Geometry check sheet. Reference: the model listing, model coordinates, mm. A direction names the side the tool comes from. Give positions to 0.01 mm unless a question says otherwise; leave off trailing zeros. Write each loop counter-clockwise with the first axis right and the second up, starting at its lowest first coordinate (ties: lowest second). Pieces come first, ordered by that corner, then holes. Notation, with made-up numbers: (-2, -16) - (26, -16) arc R31 ccw to (26, 21) - close; hole circle Ø7 at (69, 22.5). An arc over 180 degrees is marked (long way). Use a Markdown table: item, result.
```python
from build123d import *

# Parameters (mm, degrees)
SKETCH_1_R      = 20.5
EXTRUDE_1_DEPTH = 20
SKETCH_4_R      = 20
EXTRUDE_4_DEPTH = 28
SKETCH_2_R      = 11
EXTRUDE_2_DEPTH = 6
SKETCH_3_R      = 40
EXTRUDE_3_DEPTH = 5


with BuildPart() as part:
    # 草图1 → 凸台-拉伸1 (new body)
    with BuildSketch(Plane.XY):
        Circle(SKETCH_1_R)
    extrude(amount=EXTRUDE_1_DEPTH)

    # 草图4 → 凸台-拉伸4 (add)
    with BuildSketch(Plane.XY.offset(20)):
        Circle(SKETCH_4_R)
    extrude(amount=EXTRUDE_4_DEPTH)

    # 草图2 → 凸台-拉伸2 (add)
    with BuildSketch(Plane.XY.offset(48)):
        Circle(SKETCH_2_R)
    extrude(amount=EXTRUDE_2_DEPTH)

    # 草图3 → 凸台-拉伸3 (add)
    with BuildSketch(Plane.XY.offset(54)):
        Circle(SKETCH_3_R)
        with BuildLine():
            Line((-2.5, 12.247448714), (-2.5, 29.895651858))
            ThreePointArc((-2.5, 29.895651858), (-25.980762114, 15), (-27.140393972, -12.782762419))
            Line((-27.140393972, -12.782762419), (-11.856601718, -3.958660847))
            ThreePointArc((-11.856601718, -3.958660847), (-10.825317547, 6.25), (-2.5, 12.247448714))
        make_face(mode=Mode.SUBTRACT)
        with BuildLine():
            Line((11.856601718, -3.958660847), (27.140393972, -12.782762419))
            ThreePointArc((27.140393972, -12.782762419), (25.980762114, 15), (2.5, 29.895651858))
            Line((2.5, 29.895651858), (2.5, 12.247448714))
            ThreePointArc((2.5, 12.247448714), (10.825317547, 6.25), (11.856601718, -3.958660847))
        make_face(mode=Mode.SUBTRACT)
        with BuildLine():
            Line((9.356601718, -8.288787866), (24.640393972, -17.112889438))
            ThreePointArc((24.640393972, -17.112889438), (0, -30), (-24.640393972, -17.112889438))
            Line((-24.640393972, -17.112889438), (-9.356601718, -8.288787866))
            ThreePointArc((-9.356601718, -8.288787866), (0, -12.5), (9.356601718, -8.288787866))
        make_face(mode=Mode.SUBTRACT)
    extrude(amount=EXTRUDE_3_DEPTH)


solid = part.part
```
1) Depth check by flat-ended pin: P1, Ø4, axis at y = 17, z = 56.5, coming from the +X side; P2, Ø4, axis at y = 20.5, z = 55.5, coming from the -X side; P3, Ø1.5, axis at y = 6.5, z = 13.5, coming from the -X side. Enter the tip coordinate at first touch or a pass-through.
Working result:
| item | result |
|---|---|
| P1 | stops at x = 37.08 |
| P2 | stops at x = -35.46 |
| P3 | stops at x = -19.68 |
2) Section check A-A on y = 0. Record the boundary of the cut face in (x, z).
Working result:
| item | result |
|---|---|
| outline | (-40, 54) - (-30, 54) - (-30, 59) - (-40, 59) - close; (-20.5, 0) - (20.5, 0) - (20.5, 20) - (20, 20) - (20, 48) - (11, 48) - (11, 54) - (12.5, 54) - (12.5, 59) - (-12.5, 59) - (-12.5, 54) - (-11, 54) - (-11, 48) - (-20, 48) - (-20, 20) - (-20.5, 20) - close; (30, 54) - (40, 54) - (40, 59) - (30, 59) - close |
3) Section check C-C on y = -23. Record the boundary of the cut face in (x, z).
Working result:
| item | result |
|---|---|
| outline | (-32.73, 54) - (-19.26, 54) - (-19.26, 59) - (-32.73, 59) - close; (19.26, 54) - (32.73, 54) - (32.73, 59) - (19.26, 59) - close |
4) Section check D-D on x = -18. Record the boundary of the cut face in (y, z), then the cut area to 3 significant figures.
Working result:
| item | result |
|---|---|
| outline | (-35.72, 54) - (-24, 54) - (-24, 59) - (-35.72, 59) - close; (-13.28, 54) - (-7.51, 54) - (-7.51, 59) - (-13.28, 59) - close; (-9.81, 0) - (9.81, 0) - (9.81, 20) - (8.72, 20) - (8.72, 48) - (-8.72, 48) - (-8.72, 20) - (-9.81, 20) - close; (24, 54) - (35.72, 54) - (35.72, 59) - (24, 59) - close |
| area | 1,030 mm² |
5) Set-up check for faces 1 (the flat face through (8, -8, 54)), 2 (the flat face through (-1, 1, 59)), 3 (the cylindrical face through (26.18, 14.65, 56.46)), 4 (the flat face through (19.39, -8.31, 56.46)): record each of +Z, -Z, +X, -X, +Y, -Y from which the full face is reachable in a straight line by a thin tool's end or side.
Working result:
| item | result |
|---|---|
| face 1 | none |
| face 2 | +Z, +X, -X, +Y, -Y |
| face 3 | +Z, -Z |
| face 4 | +Z |
6) Material ranges on L1, parallel to Y at x = -11.5, z = 56; L2, parallel to Z at x = 9.5, y = 36; L3, parallel to Y at x = 0, z = 27.5, recorded low to high. Write a range as from..to.
Working result:
| item | result |
|---|---|
| L1 | y = -38.31..-27.71, -9.53..4.9, 27.71..38.31 |
| L2 | z = 54..59 |
| L3 | y = -20..20 |
7) Mould release check, pull along Y, two halves, no side actions. Record for faces 5 (the flat face through (-17.105, -12.763, 56.465)), 6 (the flat face through (-2.5, 21, 56)), 7 (the cylindrical face through (-2.38, -10.74, 50.96)), 8 (the flat face through (0, 0, 0)): pulls with the +Y half, pulls with the -Y half, needs draft (parallel to the pull), parting line crosses it, or undercut.
Working result:
| item | result |
|---|---|
| face 5 | undercut |
| face 6 | undercut |
| face 7 | parting line crosses it |
| face 8 | needs draft |
8) Section check B-B on x = 0. Record the boundary of the cut face in (y, z).
Working result:
| item | result |
|---|---|
| outline | (-40, 54) - (-30, 54) - (-30, 59) - (-40, 59) - close; (-20.5, 0) - (20.5, 0) - (20.5, 20) - (20, 20) - (20, 48) - (11, 48) - (11, 54) - (40, 54) - (40, 59) - (-12.5, 59) - (-12.5, 54) - (-11, 54) - (-11, 48) - (-20, 48) - (-20, 20) - (-20.5, 20) - close |
